Check sheet for the modelled part. Datum: model origin and axes. Units: mm. Face numbers are marked on the shaded views. A direction names the side the tool comes from. Give positions to 0.01 mm unless a question says otherwise; leave off trailing zeros. Write each loop counter-clockwise with the first axis right and the second up, starting at its lowest first coordinate (ties: lowest second). Pieces come first, ordered by that corner, then holes. Notation, with made-up numbers: (12.25, 52) -> (57.25, 52) arc R31 cw to (57.25, 79) -> close; hole circle Ø2 at (62.5, 59.25). An arc over 180 degrees is marked (long way). Use a Markdown table: item, result. Add a question column.
1. Cross-section at B-B (x = 15.5). Enter the section's corners in (y, z).
2. Gauge pin test, flat ends, axial feed: P1, Ø0.8, axis at y = -7.5, z = 0.5, coming from the +X side; P2, Ø6, axis at x = 5, y = -8.5, coming from the +Z side; P3, Ø1, axis at y = -6, z = 0, coming from the -X side. Record the tip position at first contact, or that the pin passes through.
3. Cross-section at A-A (y = -3). Enter the section's corners in (x, z).
4. Cross-section at C-C (z = -2.5). Enter the section's corners in (x, y).
5. Set-up check for the marked faces 1, 2 and 3: record each of +Z, -Z, +X, -X, +Y, -Y from which the full face is reachable in a straight line by a thin tool's end or side.
6. Scan lines: probe 1 along Z at (x, y) = (11, -2.25); probe 2 along Y at (x, z) = (21.75, 5); probe 3 along Z at (x, y) = (16, -2.75). Record each from-to range of solid material in increasing order. Write a range as [from, to].
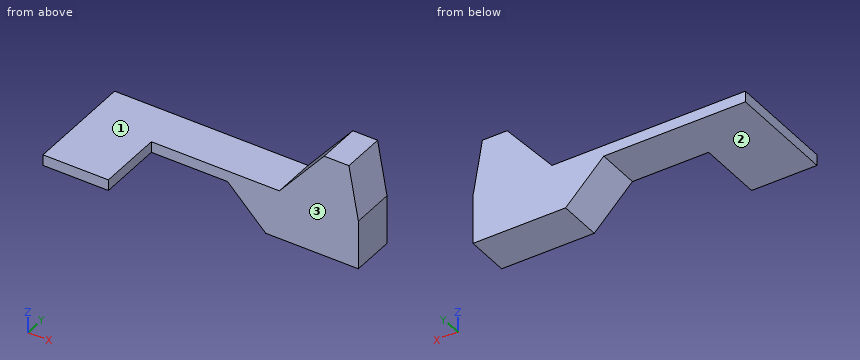
Autodesk Inventor part; units mm, degrees
ref_plane "YZ Plane" through (0, 0, 0) normal (1, 0, 0) x (0, 1, 0)
ref_plane "XZ Plane" through (0, 0, 0) normal (0, 1, 0) x (-1, 0, 0)
ref_plane "XY Plane" through (0, 0, 0) normal (0, 0, 1) x (1, 0, 0)
sketch "草圖1" plane through (0, 0, 0) normal (0, 0, 1) x (1, 0, 0)
  line L0 (0, 0) -> (25, 0)
  line L1 (25, 0) -> (25, -10)
  line L2 (25, -10) -> (0, -10)
  line L3 (0, -10) -> (0, 0)
  line L4 (25, 0) -> (7, 0)
  line L5 (7, 0) -> (7, -4)
  line L6 (7, -4) -> (25, -4)
  line L7 (25, -4) -> (25, 0)
  line L8 (26, -5) -> (6, -5)
  line L9 (6, -5) -> (6, 1)
  line L10 (6, 1) -> (26, 1)
  line L11 (26, 1) -> (26, -5)
  line L12 (7, -4) -> (6, -4)
  line L13 (6, -5) -> (6, -10)
  point P0 (25, -5)
  dimension "d0" = 25
  dimension "d1" = 10
  dimension "d2" = 18
  dimension "d3" = 4
  dimension "d4" = 1
extrude "擠出1" add sketch "草圖1" along normal blind 1 contours L5 L12 L9 L0 | L0 L1 L6 L5 | L9 L13 L2 L3 L0
sketch "草圖2" plane through (0, 0, 0) normal (0, 1, 0) x (1, 0, 0)
  line L0 (25, -1) -> (0, -1)
  line L1 (25, -1) -> (24.136, -5.9)
  line L2 (24.136, -5.9) -> (21.864, -5.9)
  line L3 (21.864, -5.9) -> (17.7524, -1)
  point P0 (0, 0)
  point P1 (23, -5.9)
  dimension "d7" = 4.9
  dimension "d8" = 2
  dimension "d9" = 80
  dimension "d10" = 50
extrude "擠出2" add sketch "草圖2" against normal up to surface (4 mm away)
sketch "草圖3" plane through (0, 0, 0) normal (0, 1, 0) x (1, 0, 0)
  line L0 (25, 0) -> (0, 0)
  line L1 (0, 0) -> (0, -1)
  line L2 (17.7524, -1) -> (0, -1)
  line L3 (17.7524, -1) -> (21.864, -5.9)
  line L4 (21.864, -5.9) -> (24.136, -5.9)
  line L5 (24.136, -5.9) -> (25, -1)
  line L6 (25, 0) -> (25, -1)
  line L7 (25, 0) -> (25, 3.5)
  line L8 (25, 3.5) -> (16.5, 3.5)
  line L9 (16.5, 3.5) -> (13, 0)
  dimension "d13" = 12
  dimension "d14" = 45
  dimension "d15" = 3.5
extrude "擠出3" add sketch "草圖3" against normal up to surface (4 mm away) contours L0 L9 L8 L7
properties part number "botton_3D 列印"
Worked answers:
| question | item | result |
|---|---|---|
| 1 | outline | (-4, -2.5) -> (0, -2.5) -> (0, 1) -> (-4, 1) -> close |
| 2 | P1 | stops at x = 6 |
| 2 | P2 | stops at z = 1 |
| 2 | P3 | stops at x = 0 |
| 3 | outline | (0, 0) -> (13, 0) -> (16.5, -3.5) -> (25, -3.5) -> (25, 1) -> (24.14, 5.9) -> (21.86, 5.9) -> (17.75, 1) -> (0, 1) -> close |
| 4 | outline | (15.5, -4) -> (25, -4) -> (25, 0) -> (15.5, 0) -> close |
| 5 | face 1 | +Z, -X, +Y, -Y |
| 5 | face 2 | -Z, -X, +Y, -Y |
| 5 | face 3 | +Z, -Z, +X, -Y |
| 6 | probe 1 | z = [0, 1] |
| 6 | probe 2 | y = [-4, 0] |
| 6 | probe 3 | z = [-3, 1] |
